from build123d import *

# Parameters (mm, degrees)
SKETCH136_R          = 2.25
SKETCH136_R_2        = 3
PAD082_DEPTH         = 30
POCKET029_DEPTH      = 28
SKETCH138_W          = 11.5
SKETCH138_H          = 28
POCKET030_DEPTH      = 15.001
POCKET030_DEPTH_BACK = 15.001


with BuildPart() as part:
    # Sketch136 → Pad082 (new body)
    with BuildSketch(Plane.XY):
        with BuildLine():
            Line((-9, -5), (9, -5))
            ThreePointArc((9, -5), (12.535534, -3.535534), (14, 0))
            Line((15, 0), (14, 0))
            Line((15, 0), (15, 10.5))
            Line((-15, 10.5), (15, 10.5))
            Line((-15, 0), (-15, 10.5))
            Line((-15, 0), (-14, 0))
            ThreePointArc((-14, 0), (-12.535534, -3.535534), (-9, -5))
        make_face()
        with Locations((-9, 0)):
            Circle(SKETCH136_R, mode=Mode.SUBTRACT)
        with Locations((9, 0)):
            Circle(SKETCH136_R, mode=Mode.SUBTRACT)
        Circle(SKETCH136_R_2, mode=Mode.SUBTRACT)
    extrude(amount=-PAD082_DEPTH)

    # Sketch137 → Pocket029 (cut)
    with BuildSketch(Plane.XY):
        Polygon((-12, 10.5), (-12, 9.5), (-13.5, 9.5), (-13.5, 8), (13.5, 8), (13.5, 9.5), (12, 9.5), (12, 10.5), align=None)
    extrude(amount=-POCKET029_DEPTH, mode=Mode.SUBTRACT)

    # Sketch138 → Pocket030 (cut, two sides)
    with BuildSketch(Plane.YZ) as pocket030_sk:
        with Locations((0.75, -16)):
            Rectangle(SKETCH138_W, SKETCH138_H)
    extrude(amount=-POCKET030_DEPTH, mode=Mode.SUBTRACT)
    extrude(pocket030_sk.sketch, amount=POCKET030_DEPTH_BACK, mode=Mode.SUBTRACT)


with BuildPart() as part_1:
    # Body119 placement: moved
    add(part.part.moved(Location((0, 32, -2))))


solid = part_1.part
Work out the finished part from the listing and answer in its coordinate system (mm). A direction names the side the tool comes from. Give positions to 0.01 mm unless a question says otherwise; leave off trailing zeros. Loops run counter-clockwise (first coordinate to the right, second up) from the corner with the lowest first, then second, coordinate; pieces in that order, holes last. Notation, with made-up numbers: (22.25, 59) - (51.25, 59) arc R30 ccw to (51.25, 83) - close; hole circle Ø5 at (-24, 43). An arc over 180 degrees is marked (long way). Answer in a Markdown table with one row per item. Add a question column.
Q1. A tool of negligible diameter and unlimited length cuts with its end or side. For faces 1 (the flat face through (-12, 42, -16)), 2 (the flat face through (-14.5, 32, -3)), 3 (the flat face through (0, 38.5, -18)), 4 (the flat face through (14.5, 32, -3)), 5 (the flat face through (-13.5, 41, -16)), from which of +Z, -Z, +X, -X, +Y, -Y can it reach the whole face along a straight path? Write none if from no direction.
Q2. The part is cut by section B-B (z = -8.5). Determine the outline of the cut face in (x, y).
Q3. The part is cut by section A-A (x = 0). Determine the outline of the cut face in (y, z), and give its area (3 significant figures).
Q4. The part is cut by section D-D (y = 33). Determine the outline of the cut face in (x, z), and give its area (3 significant figures).
Q5. Consider line 1 along Y through (x, z) = (-12.5, -13.5); line 2 along Y through (x, z) = (-9, -3.25); line 3 along Y through (x, z) = (-1.5, -23.75). Determine where each line is inside the solid, lowest interval first.
Q6. The part is cut by section C-C (x = 13). Determine the outline of the cut face in (y, z), and give its area (3 significant figures).
Q7. Each of these flat-tipped pins is pushed along its axis until it touches: P1, Ø7, axis at x = -9, y = 32, coming from the +Z side; P2, Ø2, axis at y = 36.5, z = -12, coming from the -X side; P3, Ø0.5, axis at x = 14.5, z = -3.5, coming from the -Y side; P4, Ø0.8, axis at x = -13, z = -16, coming from the -Y side. Where does it stop, or does it pass through?
Solution:
| question | item | result |
|---|---|---|
| 1 | face 1 | +Z, +Y |
| 1 | face 2 | +Z, -Z, -X, -Y |
| 1 | face 3 | -Z, +X, -X, -Y |
| 1 | face 4 | +Z, -Z, +X, -Y |
| 1 | face 5 | +Z |
| 2 | outline | (-15, 38.5) - (15, 38.5) - (15, 42.5) - (12, 42.5) - (12, 41.5) - (13.5, 41.5) - (13.5, 40) - (-13.5, 40) - (-13.5, 41.5) - (-12, 41.5) - (-12, 42.5) - (-15, 42.5) - close |
| 3 | outline | (27, -4) - (29, -4) - (29, -2) - (27, -2) - close; (35, -4) - (38.5, -4) - (38.5, -32) - (42.5, -32) - (42.5, -30) - (40, -30) - (40, -2) - (35, -2) - close |
| 3 | area | 61.0 mm² |
| 4 | outline | (-15, -4) - (-11.02, -4) - (-11.02, -2) - (-15, -2) - close; (-6.98, -4) - (-2.83, -4) - (-2.83, -2) - (-6.98, -2) - close; (2.83, -4) - (6.98, -4) - (6.98, -2) - (2.83, -2) - close; (11.02, -4) - (15, -4) - (15, -2) - (11.02, -2) - close |
| 4 | area | 32.6 mm² |
| 5 | line 1 | y = 38.5 to 40, 41.5 to 42.5 |
| 5 | line 2 | y = 27 to 29.75, 34.25 to 40 |
| 5 | line 3 | y = 38.5 to 40 |
| 6 | outline | (29, -4) - (38.5, -4) - (38.5, -32) - (42.5, -32) - (42.5, -2) - (41.5, -2) - (41.5, -30) - (40, -30) - (40, -2) - (29, -2) - close |
| 6 | area | 97.0 mm² |
| 7 | P1 | stops at z = -2 |
| 7 | P2 | passes through |
| 7 | P3 | stops at y = 32 |
| 7 | P4 | stops at y = 38.5 |
